```python
from build123d import *

# Parameters (mm, degrees)
SKETCH1_W           = 68.6
SKETCH1_H           = 53.3
BOSS_EXTRUDE1_DEPTH = 1.75
SKETCH2_R           = 1.6
CUT_EXTRUDE1_DEPTH  = 2.75
CUT_EXTRUDE2_DEPTH  = 2.75


with BuildPart() as part:
    # Sketch1 → Boss-Extrude1 (new body)
    with BuildSketch(Plane.XY):
        Rectangle(SKETCH1_W, SKETCH1_H)
    extrude(amount=BOSS_EXTRUDE1_DEPTH)

    # Sketch2 → Cut-Extrude1 (cut, through all)
    with BuildSketch(Plane.XY.offset(1.75)):
        with Locations((-19, 24.05)):
            Circle(SKETCH2_R)
        with Locations((-20.3, -24.15)):
            Circle(SKETCH2_R)
        with Locations((31.8, 8.85)):
            Circle(SKETCH2_R)
        with Locations((31.8, -19.05)):
            Circle(SKETCH2_R)
    extrude(amount=-CUT_EXTRUDE1_DEPTH, mode=Mode.SUBTRACT)

    # Sketch3 → Cut-Extrude2 (cut, through all)
    with BuildSketch(Plane.XY.offset(1.75)):
        Polygon((31.8, 26.65), (31.8, 13.85), (50.94988261, -5.29988261), (28.344966041, -27.904799179), (59.308885604, -27.904799179), (59.308885604, 26.65), align=None)
    extrude(amount=-CUT_EXTRUDE2_DEPTH, mode=Mode.SUBTRACT)


solid = part.part
```
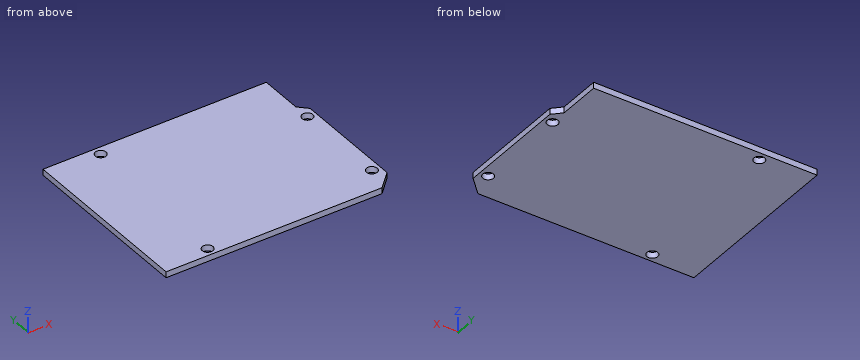
Here's how the part is built. I have some questions about the finished solid (model axes, mm). Coordinates: 2 decimals unless noted, no trailing zeros. Loops run counter-clockwise (first coordinate to the right, second up) from the corner with the lowest first, then second, coordinate; pieces in that order, holes last. Notation, with made-up numbers: (-10.75, -7.75) - (39.25, -7.75) arc R11 ccw to (39.25, 3.25) - close; hole circle Ø11 at (-2.5, -36.75). An arc over 180 degrees is marked (long way). Answer as CSV lines item,"result".
Q1. For pin 1 (0.9 mm diameter, centred on y = 18.5, z = 1, fed in from +X), with a flat end and sliding along its axis, tell me the tip position at first contact or that it passes through.
Response:
pin 1,"x = 31.8"
Q2. If we section it at B-B, the plane z = 0.3: Write out the boundary of the cut face in (x, y), and give its area (3 significant figures).
Response:
outline,"(-34.3, -26.65) - (29.6, -26.65) - (34.3, -21.95) - (34.3, 11.35) - (31.8, 13.85) - (31.8, 26.65) - (-34.3, 26.65) - close; hole circle Ø3.2 at (-20.3, -24.15); hole circle Ø3.2 at (-19, 24.05); hole circle Ø3.2 at (31.8, -19.05); hole circle Ø3.2 at (31.8, 8.85)"
area,"3,580 mm2"
Q3. If we section it at C-C, the plane y = 24.05: Write out the boundary of the cut face in (x, z), and give its area (3 significant figures).
Response:
outline,"(-34.3, 0) - (-20.6, 0) - (-20.6, 1.75) - (-34.3, 1.75) - close; (-17.4, 0) - (31.8, 0) - (31.8, 1.75) - (-17.4, 1.75) - close"
area,"110 mm2"
Q4. If we section it at A-A, the plane y = 8.85: Write out the boundary of the cut face in (x, z), and give its area (3 significant figures).
Response:
outline,"(-34.3, 0) - (30.2, 0) - (30.2, 1.75) - (-34.3, 1.75) - close; (33.4, 0) - (34.3, 0) - (34.3, 1.75) - (33.4, 1.75) - close"
area,"114 mm2"
Q5. If I drill on L1, parallel to X at y = 9, z = 0.5; L2, parallel to Y at x = -20.3, z = 0.5; L3, parallel to Y at x = -19, z = 0.6, over which ranges is the centre line in solid material (lowest first)? Write a range as [from, to].
Response:
L1,"[-34.3, 30.21], [33.39, 34.3]"
L2,"[-26.65, -25.75], [-22.55, 23.12], [24.98, 26.65]"
L3,"[-26.65, -25.08], [-23.22, 22.45], [25.65, 26.65]"
